```python
from build123d import *

# Parameters (mm, degrees)
SKETCH_W             = 101.6
SKETCH_H             = 101.6
PAD_DEPTH            = 1371.6
FILLET_R             = 19.05
SKETCH001_W          = 88.9
SKETCH001_H          = 88.9
POCKET_DEPTH         = 1371.601
FILLET001_R          = 12.7
BODY_ROLL_ANGLE      = -90
BODY_PLACEMENT_ANGLE = -90


with BuildPart() as part:
    # Sketch → Pad (new body)
    with BuildSketch(Plane.YZ):
        Rectangle(SKETCH_W, SKETCH_H)
    extrude(amount=PAD_DEPTH)

    # Fillet
    fillet_edges = [part.edges().sort_by_distance(p)[0] for p in [
        (685.8, 50.8, 50.8),
        (685.8, -50.8, 50.8),
        (685.8, 50.8, -50.8),
        (685.8, -50.8, -50.8),
    ]]
    fillet(fillet_edges, radius=FILLET_R)

    # Sketch001 → Pocket (cut, through all)
    with BuildSketch(Plane.YZ):
        Rectangle(SKETCH001_W, SKETCH001_H)
    extrude(amount=POCKET_DEPTH, mode=Mode.SUBTRACT)

    # Fillet001
    fillet001_edges = [part.edges().sort_by_distance(p)[0] for p in [
        (685.8, -44.45, -44.45),
        (685.8, -44.45, 44.45),
        (685.8, 44.45, 44.45),
        (685.8, 44.45, -44.45),
    ]]
    fillet(fillet001_edges, radius=FILLET001_R)


with BuildPart() as part_1:
    # Body roll: moved
    add(part.part.rotate(Axis((0, 0, 0), (1, 0, 0)), BODY_ROLL_ANGLE))


with BuildPart() as part_2:
    # Body placement: moved
    add(part_1.part.rotate(Axis((0, 0, 0), (0, 0, 1)), BODY_PLACEMENT_ANGLE))


solid = part_2.part
```
Can you work these out from the model? Positions are in its coordinate system, mm. A direction names the side the tool comes from. Round coordinates to 2 decimals unless told otherwise and drop trailing zeros. Loops run counter-clockwise (first coordinate to the right, second up) from the corner with the lowest first, then second, coordinate; pieces in that order, holes last. Notation, with made-up numbers: (54, 42.25) -> (82, 42.25) arc R7 ccw to (82, 53.25) -> close; hole circle Ø6 at (-32.5, 7). An arc over 180 degrees is marked (long way). Answer in a Markdown table with one row per item.
Item 1: Will these pins go through, and if not, where does the flat tip stop? P1, Ø5, axis at x = 32, y = -354, coming from the +Z side; P2, Ø4, axis at y = -502, z = 34.5, coming from the -X side; P3, Ø4, axis at y = -1170, z = 38, coming from the -X side.
Answer block:
| item | result |
|---|---|
| P1 | z = 50.8 |
| P2 | x = -50.79 |
| P3 | x = -50.32 |
Item 2: We'd pull the mould along Z, two halves only. Please class faces 3 (the flat face through (50.8, -676, 0)), 4 (the flat face through (0, -676, 50.8)), 5 (the flat face through (0, -676, -44.45)): released by +Z, released by -Z, zero draft, split by the parting line, or undercut.
Answer block:
| item | result |
|---|---|
| face 3 | zero draft |
| face 4 | released by +Z |
| face 5 | undercut |
Item 3: If I drill on probe 1 along X at (y, z) = (-1187, -23); probe 2 along X at (y, z) = (-681, -33), over which ranges is the centre line in solid material (lowest first)?
Answer block:
| item | result |
|---|---|
| probe 1 | -50.8 to -44.45, 44.45 to 50.8 |
| probe 2 | -50.76 to -44.39, 44.39 to 50.76 |
Item 4: Suppose I cut it at C-C, the plane z = 0.5. List the corners of the cut face in (x, y) for me.
Answer block:
| item | result |
|---|---|
| outline | (-50.8, -1371.6) -> (-44.45, -1371.6) -> (-44.45, 0) -> (-50.8, 0) -> close; (44.45, -1371.6) -> (50.8, -1371.6) -> (50.8, 0) -> (44.45, 0) -> close |
Item 5: Suppose I cut it at B-B, the plane x = -19. List the corners of the cut face in (y, z) for me.
Answer block:
| item | result |
|---|---|
| outline | (-1371.6, -50.8) -> (0, -50.8) -> (0, -44.45) -> (-1371.6, -44.45) -> close; (-1371.6, 44.45) -> (0, 44.45) -> (0, 50.8) -> (-1371.6, 50.8) -> close |
Item 6: Suppose I cut it at A-A, the plane y = -650.5. List the corners of the cut face in (x, z) for me.
Answer block:
| item | result |
|---|---|
| outline | (-50.8, -31.75) arc R19.05 ccw to (-31.75, -50.8) -> (31.75, -50.8) arc R19.05 ccw to (50.8, -31.75) -> (50.8, 31.75) arc R19.05 ccw to (31.75, 50.8) -> (-31.75, 50.8) arc R19.05 ccw to (-50.8, 31.75) -> close; hole (-44.45, -31.75) arc R12.7 ccw to (-31.75, -44.45) -> (31.75, -44.45) arc R12.7 ccw to (44.45, -31.75) -> (44.45, 31.75) arc R12.7 ccw to (31.75, 44.45) -> (-31.75, 44.45) arc R12.7 ccw to (-44.45, 31.75) -> close |
Item 7: On a 3-axis mill with a long thin cutter (end or side, diameter ignored), from which of +Z, -Z, +X, -X, +Y, -Y can I reach the whole of each face in a straight line? I mean faces 1 (the flat face through (-50.8, -676, 0)), 2 (the flat face through (0, -676, 44.45)). Say none if no direction works.
Answer block:
| item | result |
|---|---|
| face 1 | +Z, -Z, -X, +Y, -Y |
| face 2 | +Y, -Y |
